Verification items for this drawing (mm, ordinates from the low corner). Round coordinates to 2 decimals unless told otherwise and drop trailing zeros. Loops run counter-clockwise (first coordinate to the right, second up) from the corner with the lowest first, then second, coordinate; pieces in that order, holes last. Notation, with made-up numbers: (5, 34) -> (59, 34) arc R16 ccw to (59, 42) -> close; hole circle Ø3 at (70.25, 72). An arc over 180 degrees is marked (long way). One line per question, with ' | ' between items.
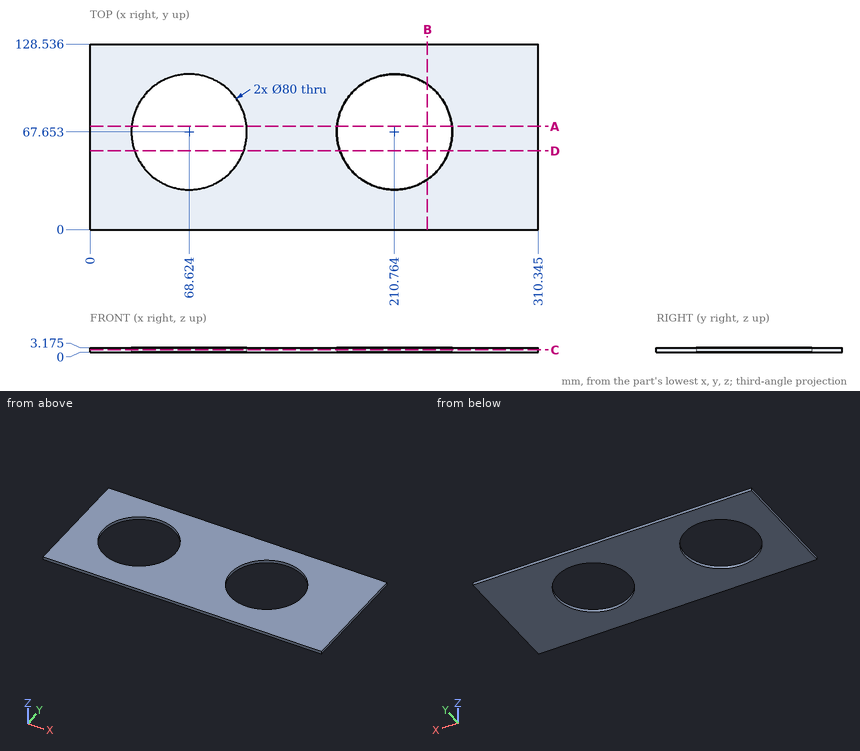
(1) Sectioned sample at A-A, the plane y = 71.5. Record the cut outline in (x, z) (1 decimal).
Answer:
outline: (0, 0) -> (28.8, 0) -> (28.8, 3.2) -> (0, 3.2) -> close; (108.4, 0) -> (170.9, 0) -> (170.9, 3.2) -> (108.4, 3.2) -> close; (250.6, 0) -> (310.3, 0) -> (310.3, 3.2) -> (250.6, 3.2) -> close
(2) Sectioned sample at D-D, the plane y = 54.5. Record the cut outline in (x, z) (1 decimal).
Answer:
outline: (0, 0) -> (30.8, 0) -> (30.8, 3.2) -> (0, 3.2) -> close; (106.4, 0) -> (173, 0) -> (173, 3.2) -> (106.4, 3.2) -> close; (248.5, 0) -> (310.3, 0) -> (310.3, 3.2) -> (248.5, 3.2) -> close
(3) Sectioned sample at C-C, the plane z = 1.7. Record the cut outline in (x, y) (1 decimal), and give its area (3 significant figures).
Answer:
outline: (0, 0) -> (310.3, 0) -> (310.3, 128.5) -> (0, 128.5) -> close; hole circle Ø80 at (68.6, 67.7); hole circle Ø80 at (210.8, 67.7) | area: 29,800 mm2
(4) Scan lines: probe 1 along X at (y, z) = (66, 1.55) (1 decimal); probe 2 along X at (y, z) = (82.5, 0.35) (1 decimal); probe 3 along Y at (x, z) = (222, 3.05) (1 decimal). Record each from-to range of solid material in increasing order.
Answer:
probe 1: x = 0 to 28.7, 108.6 to 170.8, 250.7 to 310.3 | probe 2: x = 0 to 31.5, 105.8 to 173.6, 247.9 to 310.3 | probe 3: y = 0 to 29.3, 106 to 128.5
(5) Sectioned sample at B-B, the plane x = 233.5. Record the cut outline in (y, z) (1 decimal), and give its area (3 significant figures).
Answer:
outline: (0, 0) -> (34.7, 0) -> (34.7, 3.2) -> (0, 3.2) -> close; (100.6, 0) -> (128.5, 0) -> (128.5, 3.2) -> (100.6, 3.2) -> close | area: 199 mm2
